```python
from build123d import *

# Parameters (mm, degrees)
F0_W        = 101.2
F0_H        = 101.2
F1_DEPTH    = 200
F2_T        = -1.2
F4_W        = 0.8
F4_H        = 0.8
F5_DEPTH    = 200.001
F6_R        = 1.2
F7_T4_DEPTH = 101.8
F8_R        = 2.4
F9_T1_DEPTH = 110.8
F12_DEPTH   = 25
F13_DEPTH   = 25
F15_DEPTH   = 25


# Not quite as in the source:
# - a fillet or chamfer that OpenCascade refuses, or shapes differently, is made with other operations: its cross-section is extruded or revolved along the edge and cut away or added


with BuildPart() as f1:
    # F0 (on Top) → F1 (new body)
    with BuildSketch(Plane.XY):
        Rectangle(F0_W, F0_H)
    extrude(amount=F1_DEPTH)

    # F2
    f2_openings = [f1.faces().sort_by_distance(p)[0] for p in [
        (0, 0, 200),
        (0, -50.6, 100),
        (50.6, 0, 100),
    ]]
    offset(amount=F2_T, openings=f2_openings)

    # F4 (on face) → F5 (cut, through all)
    with BuildSketch(Plane.XY.offset(200)):
        with Locations((-49, 49)):
            Rectangle(F4_W, F4_H)
        Polygon((-50.6, 50.6), (-50.6, 48.6), (-49.4, 48.6), (-49.4, 49.4), (-48.6, 49.4), (-48.6, 50.6), align=None)
    extrude(amount=-F5_DEPTH, mode=Mode.SUBTRACT)

    # F6
    f6_edges = [f1.edges().sort_by_distance(p)[0] for p in [
        (1, 49.4, 1.2),
    ]]
    fillet(f6_edges, radius=F6_R)

    # F7: fillet of radius 1.2 on 1 edges, made by hand


with BuildPart() as f7_tool2:
    # F7_s3 → F7_t4 (new body)
    with BuildSketch(Plane.XZ.offset(50.6)):
        with BuildLine():
            ThreePointArc((-49.4, 2.4), (-49.0485281374, 1.5514718626), (-48.2, 1.2))
            Line((-48.2, 1.2), (-49.4, 1.2))
            Line((-49.4, 1.2), (-49.4, 2.4))
        make_face()
    extrude(amount=-F7_T4_DEPTH)

    split(bisect_by=Plane.XZ.offset(-48.6), keep=Keep.TOP)


with BuildPart() as f1_1:
    add(f1.part)

    # F7_t1: union F7_tool2
    add(f7_tool2.part)

    # F8
    f8_edges = [f1_1.edges().sort_by_distance(p)[0] for p in [
        (-50.6, -1, 0),
    ]]
    fillet(f8_edges, radius=F8_R)

    # F9: fillet of radius 2.4 on 1 edges, made by hand

    # F9_s2 → F9_t1 (cut)
    with BuildSketch(Plane.YZ.offset(-54.2)):
        with BuildLine():
            ThreePointArc((50.6, 2.4), (49.8970562748, 0.7029437252), (48.2, 0))
            Line((48.2, 0), (50.6, 0))
            Line((50.6, 0), (50.6, 2.4))
        make_face()
    extrude(amount=F9_T1_DEPTH, mode=Mode.SUBTRACT)

    # F11 (on face) → F12 (cut)
    with BuildSketch(Plane(origin=(0, 50.6, 0), x_dir=(-1, 0, 0), z_dir=(0, 1, 0))):
        Polygon((-11.4, 200), (-50.6, 200), (-50.6, 30), align=None)
    extrude(amount=-F12_DEPTH, mode=Mode.SUBTRACT)

    # F10 (on face) → F13 (cut)
    with BuildSketch(Plane(origin=(-50.6, 0, 0), x_dir=(0, -1, 0), z_dir=(-1, 0, 0))):
        Polygon((50.6, 30), (50.6, 200), (11.4, 200), align=None)
    extrude(amount=-F13_DEPTH, mode=Mode.SUBTRACT)

    # F14 (on face) → F15 (cut)
    with BuildSketch(Plane(origin=(0, 0, 0), x_dir=(1, 0, 0), z_dir=(0, 0, -1))):
        Polygon((50.6, -48.2), (50.6, 50.6), (-48.2, 50.6), align=None)
    extrude(amount=-F15_DEPTH, mode=Mode.SUBTRACT)


solid = f1_1.part
```
Design review of the part built by this model. Coordinates are the model's own, in mm. A direction names the side the tool comes from. Give positions to 0.01 mm unless a question says otherwise; leave off trailing zeros. Loops run counter-clockwise (first coordinate to the right, second up) from the corner with the lowest first, then second, coordinate; pieces in that order, holes last. Notation, with made-up numbers: M 76.5,49.5 L 123.5,49.5 A9 ccw 123.5,65.5 Z; hole C 21,54 d3. An arc over 180 degrees is marked long. Return JSON: item names as keys, results as strings. Group by question number.
Item 1: Tool access review of faces 1 (the flat face through (-49.4, 9, 100)), 2 (the flat face through (-11, 49.4, 100)), 3 (the flat face through (-10, 10, 1.2)): name each direction out of +Z, -Z, +X, -X, +Y, -Y from which nothing blocks a thin tool from reaching the whole face with its end or side.
Item 2: We need section B-B (y = -9). Give the boundary of the cut face in (x, z), and give its area (3 significant figures).
Item 3: For probe 1 along X at (y, z) = (17, 120.5); probe 2 along Y at (x, z) = (4.5, 137); probe 3 along Z at (x, y) = (-19.5, 24), list the stretches that pass through material, from the lowest coordinate up.
Item 4: We need section C-C (x = -4). Give the boundary of the cut face in (y, z), and give its area (3 significant figures).
Item 5: We need section A-A (z = 168). Give the boundary of the cut face in (x, y).
Item 6: Insertion check: pin 1 Ø1.5 at (y, z) = (-26.5, 42.5) entering from +X; pin 2 Ø1.6 at (x, z) = (-50, 119) entering from +Y; pin 3 Ø6 at (x, y) = (2.5, 37.5) entering from +Z. Each pin has a flat end and moves straight along its axis. Give the tip position at first contact, or say it passes through.
Item 7: We need section D-D (z = 33.5). Give the boundary of the cut face in (x, y).
Output:
{
 "1": {"face 1": "+Z, +X, +Y, -Y", "face 2": "+Z, +X, -X, -Y", "face 3": "+Z, +X, -Y"},
 "2": {"outline": "M -50.6,2.4 A2.4 ccw -48.2,0 L -6.6,0 L -6.6,1.2 L -48.2,1.2 A1.2 cw -49.4,2.4 L -49.4,200 L -50.6,200 Z", "area": "290 mm^2"},
 "3": {"probe 1": "x = -50.6 to -49.4", "probe 2": "y = 49.4 to 50.6", "probe 3": "z = 0 to 1.2"},
 "4": {"outline": "M -6.4,0 L 48.2,0 A2.4 ccw 50.6,2.4 L 50.6,200 L 49.4,200 L 49.4,2.4 A1.2 cw 48.2,1.2 L -6.4,1.2 Z", "area": "306 mm^2"},
 "5": {"outline": "M -50.6,-18.78 L -49.4,-18.78 L -49.4,48.6 L -50.6,48.6 Z; M -48.6,49.4 L 18.78,49.4 L 18.78,50.6 L -48.6,50.6 Z"},
 "6": {"pin 1": "stops at x = -49.4", "pin 2": "stops at y = 48.6", "pin 3": "stops at z = 1.2"},
 "7": {"outline": "M -50.6,-49.79 L -49.4,-49.79 L -49.4,48.6 L -50.6,48.6 Z; M -48.6,49.4 L 49.79,49.4 L 49.79,50.6 L -48.6,50.6 Z"}
}
